CAD build for the part. Positions are in the model's coordinates, mm. Coordinates: 2 decimals unless noted, no trailing zeros. Loops run counter-clockwise (first coordinate to the right, second up) from the corner with the lowest first, then second, coordinate; pieces in that order, holes last. Notation, with made-up numbers: (-7, 62) -> (1, 62) arc R9 cw to (1, 73) -> close; hole circle Ø1 at (44, -22). An arc over 180 degrees is marked (long way). Write each question's results on one line, items separated by ' | '.
Autodesk Inventor part; units mm, degrees
ref_plane "Zplus_face" through (0, 0, 1.5875) normal (0, 0, 1) x (1, 0, 0)
ref_plane "Work Plane_ConnX" through (-32, 0, 0) normal (1, 0, 0) x (0, 1, 0)
ref_plane "Work Plane_ConnY" through (0, 0, 0) normal (0, 1, 0) x (-1, 0, 0)
sketch "AL_spacer_contact_Zminus" plane through (0, 0, 0) normal (0, 0, 1) x (1, 0, 0)
  circle A0 centre (39.5, 39.5) radius 3.175
  circle A1 centre (39.5, -39.5) radius 3.175
  circle A2 centre (-39.5, -39.5) radius 3.175
  circle A3 centre (-39.5, 39.5) radius 3.175
  point P0 (0, 0)
  dimension "d228" = 39.5
  dimension "d229" = 39.5
  dimension "d230" = 39.5
  dimension "d231" = 39.5
  dimension "d232" = 39.5
  dimension "d233" = 39.5
  dimension "d234" = 39.5
  dimension "d235" = 39.5
  dimension "d236" = 6.35
sketch "Delrin_stayout_Zminus" plane through (0, 0, 0) normal (0, 0, 1) x (1, 0, 0)
  line L0 (47.5, 39.5) -> (47.5, 31)
  line L1 (47.5, 31) -> (39.5, 31)
  line L2 (39.5, 31) -> (31, 39.5)
  line L3 (31, 39.5) -> (31, 47.5)
  line L4 (31, 47.5) -> (39.5, 47.5)
  line L5 (39.5, 47.5) -> (47.5, 39.5)
  line L6 (-39.5, 47.5) -> (-47.5, 39.5)
  line L7 (-47.5, 39.5) -> (-47.5, 31)
  line L8 (-47.5, 31) -> (-39.5, 31)
  line L9 (-39.5, 31) -> (-31, 39.5)
  line L10 (-31, 39.5) -> (-31, 47.5)
  line L11 (-31, 47.5) -> (-39.5, 47.5)
  line L12 (47.5, -39.5) -> (39.5, -47.5)
  line L13 (39.5, -47.5) -> (31, -47.5)
  line L14 (31, -47.5) -> (31, -39.5)
  line L15 (31, -39.5) -> (39.5, -31)
  line L16 (39.5, -31) -> (47.5, -31)
  line L17 (47.5, -31) -> (47.5, -39.5)
  line L18 (-39.5, -47.5) -> (-47.5, -39.5)
  line L19 (-47.5, -39.5) -> (-47.5, -31)
  line L20 (-47.5, -31) -> (-39.5, -31)
  line L21 (-39.5, -31) -> (-31, -39.5)
  line L22 (-31, -39.5) -> (-31, -47.5)
  line L23 (-31, -47.5) -> (-39.5, -47.5)
  point P0 (0, 0)
  dimension "d243" = 16.5
  dimension "d244" = 8
  dimension "d245" = 8.5
  dimension "d246" = 16.5
  dimension "d247" = 47.5
  dimension "d248" = 47.5
  dimension "d249" = 47.5
  dimension "d250" = 47.5
  dimension "d251" = 47.5
  dimension "d252" = 47.5
  dimension "d253" = 47.5
  dimension "d254" = 47.5
sketch "Nub_stayout_Zminus" plane through (0, 0, 0) normal (0, 0, 1) x (1, 0, 0)
  line L0 (29, 47.5) -> (39.5, 47.5)
  line L1 (39.5, 47.5) -> (47.5, 39.5)
  line L2 (47.5, 39.5) -> (47.5, 29)
  line L3 (47.5, 29) -> (42, 29)
  line L4 (42, 29) -> (42, 40.4125)
  line L5 (40.4125, 42) -> (29, 42)
  line L6 (29, 42) -> (29, 47.5)
  arc A0 (42, 40.4125) -> (40.4125, 42) centre (40.4125, 40.4125) ccw
  line L7 (-29, 47.5) -> (-39.5, 47.5)
  line L8 (-39.5, 47.5) -> (-47.5, 39.5)
  line L9 (-47.5, 39.5) -> (-47.5, 29)
  line L10 (-47.5, 29) -> (-42, 29)
  line L11 (-42, 29) -> (-42, 40.4125)
  line L12 (-40.4125, 42) -> (-29, 42)
  line L13 (-29, 42) -> (-29, 47.5)
  arc A1 (-40.4125, 42) -> (-42, 40.4125) centre (-40.4125, 40.4125) ccw
  line L14 (-47.5, -29) -> (-42, -29)
  line L15 (-42, -29) -> (-42, -40.4125)
  line L16 (-40.4125, -42) -> (-29, -42)
  line L17 (-29, -42) -> (-29, -47.5)
  line L18 (-29, -47.5) -> (-39.5, -47.5)
  line L19 (-39.5, -47.5) -> (-47.5, -39.5)
  line L20 (-47.5, -39.5) -> (-47.5, -29)
  arc A2 (-42, -40.4125) -> (-40.4125, -42) centre (-40.4125, -40.4125) ccw
  line L21 (47.5, -29) -> (42, -29)
  line L22 (42, -29) -> (42, -40.4125)
  line L23 (40.4125, -42) -> (29, -42)
  line L24 (29, -42) -> (29, -47.5)
  line L25 (29, -47.5) -> (39.5, -47.5)
  line L26 (39.5, -47.5) -> (47.5, -39.5)
  line L27 (47.5, -39.5) -> (47.5, -29)
  arc A3 (40.4125, -42) -> (42, -40.4125) centre (40.4125, -40.4125) ccw
  point P0 (0, 0)
  dimension "d255" = 1.5875
  dimension "d256" = 18.5
  dimension "d257" = 8
  dimension "d258" = 5.5
  dimension "d259" = 47.5
  dimension "d260" = 47.5
  dimension "d264" = 1.5875
  dimension "d265" = 47.5
  dimension "d266" = 47.5
  dimension "d267" = 1.5875
  dimension "d268" = 47.5
  dimension "d269" = 47.5
  dimension "d270" = 1.5875
  dimension "d271" = 47.5
  dimension "d272" = 47.5
ref_plane "Zplus_face" through (0, 0, 1.5875) normal (0, 0, 1) x (1, 0, 0)
sketch "AL_spacer_contact_Zplus" plane through (0, 0, 1.5875) normal (0, 0, 1) x (1, 0, 0)
  circle A0 centre (-39.5, 39.5) radius 3.175
  circle A1 centre (-39.5, -39.5) radius 3.175
  circle A2 centre (39.5, -39.5) radius 3.175
  circle A3 centre (39.5, 39.5) radius 3.175
  point P0 (0, 0)
  dimension "d129" = 39.5
  dimension "d130" = 39.5
  dimension "d131" = 39.5
  dimension "d132" = 39.5
  dimension "d133" = 6.35
sketch "Delrin_stayout_Zplus" plane through (0, 0, 1.5875) normal (0, 0, 1) x (1, 0, 0)
  line L0 (47.5, -31) -> (47.5, -39.5)
  line L1 (47.5, -39.5) -> (39.5, -47.5)
  line L2 (39.5, -47.5) -> (31, -47.5)
  line L3 (31, -47.5) -> (31, -39.5)
  line L4 (31, -39.5) -> (39.5, -31)
  line L5 (39.5, -31) -> (47.5, -31)
  line L6 (47.5, 31) -> (47.5, 39.5)
  line L7 (47.5, 39.5) -> (39.5, 47.5)
  line L8 (39.5, 47.5) -> (31, 47.5)
  line L9 (31, 47.5) -> (31, 39.5)
  line L10 (31, 39.5) -> (39.5, 31)
  line L11 (39.5, 31) -> (47.5, 31)
  line L12 (-39.5, 47.5) -> (-47.5, 39.5)
  line L13 (-47.5, 39.5) -> (-47.5, 31)
  line L14 (-47.5, 31) -> (-39.5, 31)
  line L15 (-39.5, 31) -> (-31, 39.5)
  line L16 (-31, 39.5) -> (-31, 47.5)
  line L17 (-31, 47.5) -> (-39.5, 47.5)
  line L18 (-47.5, -39.5) -> (-39.5, -47.5)
  line L19 (-39.5, -47.5) -> (-31, -47.5)
  line L20 (-31, -47.5) -> (-31, -39.5)
  line L21 (-31, -39.5) -> (-39.5, -31)
  line L22 (-39.5, -31) -> (-47.5, -31)
  line L23 (-47.5, -31) -> (-47.5, -39.5)
  point P0 (0, 0)
  dimension "d115" = 16.5
  dimension "d116" = 16.5
  dimension "d117" = 8
  dimension "d118" = 8.5
  dimension "d121" = 47.5
  dimension "d122" = 47.5
  dimension "d123" = 47.5
  dimension "d124" = 47.5
  dimension "d125" = 47.5
  dimension "d126" = 47.5
  dimension "d127" = 47.5
  dimension "d128" = 47.5
sketch "Nub_stayout_Zplus" plane through (0, 0, 1.5875) normal (0, 0, 1) x (1, 0, 0)
  line L0 (47.5, 29) -> (42, 29)
  line L1 (42, 29) -> (42, 40.4125)
  line L2 (40.4125, 42) -> (29, 42)
  line L3 (29, 42) -> (29, 47.5)
  arc A0 (42, 40.4125) -> (40.4125, 42) centre (40.4125, 40.4125) ccw
  line L4 (29, 47.5) -> (39.5, 47.5)
  line L5 (39.5, 47.5) -> (47.5, 39.5)
  line L6 (47.5, 39.5) -> (47.5, 29)
  line L7 (-39.5, 47.5) -> (-29, 47.5)
  line L8 (-29, 47.5) -> (-29, 42)
  line L9 (-29, 42) -> (-40.4125, 42)
  line L10 (-42, 40.4125) -> (-42, 29)
  line L11 (-42, 29) -> (-47.5, 29)
  line L12 (-47.5, 29) -> (-47.5, 39.5)
  line L13 (-47.5, 39.5) -> (-39.5, 47.5)
  arc A1 (-40.4125, 42) -> (-42, 40.4125) centre (-40.4125, 40.4125) ccw
  line L14 (-47.5, -29) -> (-47.5, -39.5)
  line L15 (-47.5, -39.5) -> (-39.5, -47.5)
  line L16 (-39.5, -47.5) -> (-29, -47.5)
  line L17 (-29, -47.5) -> (-29, -42)
  line L18 (-29, -42) -> (-40.4125, -42)
  line L19 (-42, -40.4125) -> (-42, -29)
  line L20 (-42, -29) -> (-47.5, -29)
  arc A2 (-42, -40.4125) -> (-40.4125, -42) centre (-40.4125, -40.4125) ccw
  line L21 (29, -47.5) -> (39.5, -47.5)
  line L22 (39.5, -47.5) -> (47.5, -39.5)
  line L23 (47.5, -39.5) -> (47.5, -29)
  line L24 (47.5, -29) -> (42, -29)
  line L25 (42, -29) -> (42, -40.4125)
  line L26 (40.4125, -42) -> (29, -42)
  line L27 (29, -42) -> (29, -47.5)
  arc A3 (40.4125, -42) -> (42, -40.4125) centre (40.4125, -40.4125) ccw
  point P0 (0, 0)
  dimension "d146" = 1.5875
  dimension "d147" = 5.5
  dimension "d149" = 18.5
  dimension "d150" = 8
  dimension "d151" = 47.5
  dimension "d152" = 47.5
  dimension "d153" = 1.5875
  dimension "d154" = 47.5
  dimension "d155" = 47.5
  dimension "d156" = 1.5875
  dimension "d157" = 47.5
  dimension "d158" = 47.5
  dimension "d159" = 1.5875
  dimension "d160" = 47.5
  dimension "d161" = 47.5
sketch "Sketch1" plane through (0, 0, 0) normal (0, 0, 1) x (1, 0, 0)
  line L0 (-47.5, 47.5) -> (47.5, 47.5)
  line L1 (47.5, 47.5) -> (47.5, -47.5)
  line L2 (47.5, -47.5) -> (-47.5, -47.5)
  line L3 (-47.5, -47.5) -> (-47.5, 47.5)
  point P0 (0, 0)
  dimension "d0" = 95
  dimension "d1" = 95
  dimension "d2" = 47.5
  dimension "d3" = 47.5
extrude "Extrusion1" add sketch "Sketch1" along normal blind 1.5875
chamfer "Chamfer2" distance 11 angle 45 4 edges at (-47.5, -47.5, 0.7937) (47.5, -47.5, 0.7937) (47.5, 47.5, 0.7937) (-47.5, 47.5, 0.7937)
ref_plane "Work Plane_ConnX" through (-32, 0, 0) normal (1, 0, 0) x (0, 1, 0)
ref_plane "Work Plane_ConnY" through (0, 0, 0) normal (0, 1, 0) x (-1, 0, 0)
sketch "Sketch9" plane through (0, 0, 1.5875) normal (0, 0, 1) x (1, 0, 0)
  line L0 (47.5, 47.5) -> (47.5, -47.5)
  line L1 (58.5598, -32) -> (-58.5598, -32)
  circle A0 centre (-2.667, -21.9289) radius 0.4445
  circle A1 centre (-2.667, -42.0711) radius 0.4445
  line L2 (0, 26.5598) -> (0, -90.5598) construction
  point P0 (0, 0)
  point P1 (0, -32)
  dimension "d134" = 20.1422
  dimension "d136" = 2.667
  dimension "d138" = 0.889
  dimension "d141" = 180
  dimension "d350" = 32
  dimension "d351" = 0
extrude "Holes_Conn_Zminus" cut sketch "Sketch9" against normal through all
sketch "Sketch22" plane through (0, 0, 1.5875) normal (0, 0, 1) x (1, 0, 0)
  line L0 (47.5, 36.5) -> (47.5, -36.5)
  line L1 (0, -1.0026) -> (0, -62.9974) construction
  line L2 (62.8115, -32) -> (-62.8115, -32)
  circle A0 centre (2.032, -22.7545) radius 0.4445
  circle A1 centre (2.032, -41.2455) radius 0.4445
  point P0 (0, 0)
  point P1 (0, -32)
  dimension "d282" = 180
  dimension "d283" = 18.491
  dimension "d284" = 0.889
  dimension "d285" = 2.032
  dimension "d352" = 32
  dimension "d353" = 0
extrude "Holes_Conn_Zplus" cut sketch "Sketch22" against normal through all
hole "Hole5" at (39.5, 39.5, 1.5875) direction (0, 0, -1) diameter 3.2 end through all
mirror "Mirror5" about plane through (0, 0, 0) normal (1, 0, 0) of "Hole5"
mirror "Mirror6" about plane through (0, 0, 0) normal (0, 1, 0) of "Hole5", "Mirror5"
sketch "Sketch25" plane through (0, 0, 1.5875) normal (0, 0, 1) x (1, 0, 0)
  circle A0 centre (-39.5, -39.5) radius 1.6
  circle A1 centre (39.5, -39.5) radius 1.6
  circle A2 centre (-39.5, 39.5) radius 1.6
  circle A3 centre (39.5, 39.5) radius 1.6
  line L0 (36.5, -47.5) -> (-36.5, -47.5)
  line L1 (0, 0) -> (0, -59.2198)
  line L2 (8, -47.5) -> (8, -15.5)
  line L3 (8, -15.5) -> (-8, -15.5)
  line L4 (-8, -15.5) -> (-8, -47.5)
  line L5 (-8, -47.5) -> (-62.7516, -61.7336)
  line L6 (-62.7516, -61.7336) -> (-64.2933, 68.2222)
  line L7 (-64.2933, 68.2222) -> (58.3572, 62.5728)
  line L8 (58.3572, 62.5728) -> (56.5848, -69.017)
  line L9 (56.5848, -69.017) -> (8, -47.5)
  dimension "d362" = 16
  dimension "d363" = 32
extrude "Extrusion9" [suppressed]
sketch "Sketch26" plane through (0, 0, 1.5875) normal (0, 0, 1) x (1, 0, 0)
  line L0 (36.5, -47.5) -> (-36.5, -47.5)
  circle A0 centre (16.5, -42.5) radius 0.75
  circle A1 centre (23.5, -42.5) radius 0.75
  line L1 (20, -36.5) -> (20, -45.9188)
  point P0 (0, 0)
  point P1 (20, -42.5)
  dimension "d366" = 1.5
  dimension "d367" = 7
  dimension "d368" = 5
  dimension "d369" = 20
extrude "Extrusion10" cut sketch "Sketch26" against normal through all
sketch "Sketch28" plane through (0, 0, 1.5875) normal (0, 0, 1) x (1, 0, 0)
  line L0 (-36.5, 47.5) -> (36.5, 47.5)
  line L1 (0, 0) -> (0, 18.8917)
  line L2 (-13, 47.5) -> (13, 47.5)
  line L3 (13, 47.5) -> (13, 21.5)
  line L4 (13, 21.5) -> (-13, 21.5)
  line L5 (-13, 21.5) -> (-13, 47.5)
  dimension "d372" = 26
  dimension "d373" = 26
extrude "Extrusion11" cut sketch "Sketch28" against normal through all
fillet "Fillet3" radius 0.7937 2 edges at (-13, 21.5, 0.7937) (13, 21.5, 0.7937)
sketch "Sketch29" plane through (0, 0, 1.5875) normal (0, 0, 1) x (1, 0, 0)
  line L0 (36.5, -47.5) -> (-36.5, -47.5)
  circle A0 centre (-27.5, -43) radius 1.39
  circle A1 centre (27.5, -43) radius 1.39
  arc A2 (-26.11, -47.5) -> (-28.89, -47.5) centre (-27.5, -47.5) ccw
  arc A3 (28.89, -47.5) -> (26.11, -47.5) centre (27.5, -47.5) ccw
  line L1 (0, 0) -> (0, -8.2455)
  dimension "d377" = 2.78
  dimension "d379" = 4.5
  dimension "d380" = 55
extrude "Extrusion12" [suppressed]
sketch "Sketch30" plane through (0, 0, 1.5875) normal (0, 0, 1) x (1, 0, 0)
  line L0 (-47.5, -36.5) -> (-47.5, 36.5)
  circle A0 centre (-27.5, -43) radius 1.39
  circle A1 centre (-47.5, 27.5) radius 1.39
  circle A2 centre (-47.5, -27.5) radius 1.39
  circle A3 centre (-43, -27.5) radius 1.39
  circle A4 centre (-43, 27.5) radius 1.39
  line L1 (0, 0) -> (-6.8618, 0)
  dimension "d383" = 4.5
  dimension "d384" = 55
extrude "Extrusion13" [suppressed]
sketch "Sketch31" plane through (0, 0, 1.5875) normal (0, 0, 1) x (1, 0, 0)
  line L0 (-47.5, -36.5) -> (-47.5, 36.5)
  line L1 (36.5, -47.5) -> (-36.5, -47.5)
  line L2 (47.5, 36.5) -> (47.5, -36.5)
  line L3 (13, 47.5) -> (36.5, 47.5)
  line L4 (-47.545, 47.455) -> (47.5, 47.5) construction
  line L5 (47.5, 47.5) -> (47.545, -47.455) construction
  line L6 (47.545, -47.455) -> (-47.5, -47.5) construction
  line L7 (-47.5, -47.5) -> (-47.545, 47.455) construction
  point P0 (0, 0)
decal "Decal1"
sketch "Sketch32" plane through (0, 0, 0) normal (0, 0, -1) x (-1, 0, 0)
  line L0 (-47.5, 36.5) -> (-47.5, -36.5)
  line L1 (-36.5, -47.5) -> (36.5, -47.5)
  line L2 (47.5, -36.5) -> (47.5, 36.5)
  line L3 (36.5, 47.5) -> (13, 47.5)
  line L4 (-47.545, 47.455) -> (47.5, 47.5) construction
  line L5 (47.5, 47.5) -> (47.545, -47.455) construction
  line L6 (47.545, -47.455) -> (-47.5, -47.5) construction
  line L7 (-47.5, -47.5) -> (-47.545, 47.455) construction
  point P0 (0, 0)
decal "Decal2"
properties part number "PCB_Batt1" material "FR4"
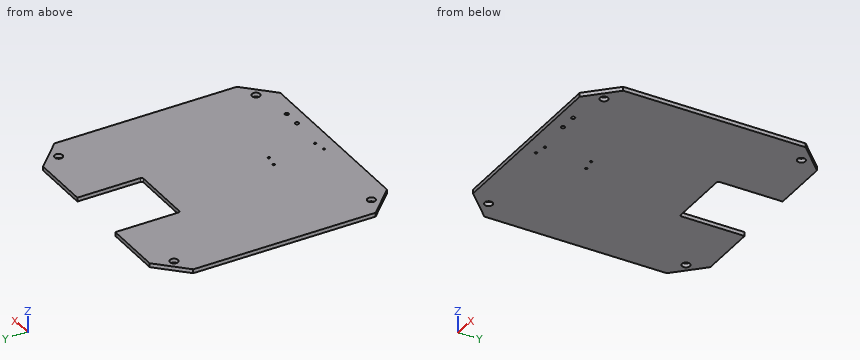
Q1. Cut at A-A on x = 39.5. Write the cut outline in (y, z).
Results are:
outline: (-44.5, 0) -> (-41.1, 0) -> (-41.1, 1.59) -> (-44.5, 1.59) -> close; (-37.9, 0) -> (37.9, 0) -> (37.9, 1.59) -> (-37.9, 1.59) -> close; (41.1, 0) -> (44.5, 0) -> (44.5, 1.59) -> (41.1, 1.59) -> close
Q2. Cut at B-B on y = 39.5. Write the cut outline in (x, z), and give its area (3 significant figures).
Results are:
outline: (-44.5, 0) -> (-41.1, 0) -> (-41.1, 1.59) -> (-44.5, 1.59) -> close; (-37.9, 0) -> (-13, 0) -> (-13, 1.59) -> (-37.9, 1.59) -> close; (13, 0) -> (37.9, 0) -> (37.9, 1.59) -> (13, 1.59) -> close; (41.1, 0) -> (44.5, 0) -> (44.5, 1.59) -> (41.1, 1.59) -> close | area: 89.9 mm^2
Q3. Wall check: L1, parallel to Y at x = 2, z = 1.25; L2, parallel to Y at x = 39.5, z = 0.7. Give the ranges that are in metal, low to high. Write a range as from..to.
Results are:
L1: -47.5..-41.69, -40.8..-23.2, -22.31..21.5 | L2: -44.5..-41.1, -37.9..37.9, 41.1..44.5
Q4. Cut at D-D on z = 0.8. Give the number of separate pieces and of enclosed holes in the cut face, and give its area (3 significant figures).
Results are:
separate pieces: 1 | enclosed holes: 10 | area: 8,070 mm^2
